```python
from build123d import *

# Parameters (mm, degrees)
F1_DEPTH = 30
F3_R     = 35
F4_DEPTH = 4
F5_D     = 9


with BuildPart() as f1:
    # F0 (on Right) → F1 (new body)
    with BuildSketch(Plane.YZ):
        with BuildLine():
            ThreePointArc((139.7, -30), (169.7, 0), (139.7, 30))
            Line((139.7, 30), (-139.7, 30))
            ThreePointArc((-139.7, 30), (-169.7, 0), (-139.7, -30))
            Line((-139.7, -30), (139.7, -30))
        make_face()
    extrude(amount=F1_DEPTH)

    # F3 (on mid) → F4 (cut, symmetric)
    with BuildSketch(Plane(origin=(15, 0, 0), x_dir=(0, -1, 0), z_dir=(-1, 0, 0))):
        with Locations((139.7, 0)):
            Circle(F3_R)
    extrude(amount=F4_DEPTH, both=True, mode=Mode.SUBTRACT)

    # F5 (through all)
    with Locations(Plane(origin=(0, 0, 0), x_dir=(0, 1, 0), z_dir=(-1, 0, 0))):
        with Locations((-139.7, 0)):
            Hole(F5_D / 2)


solid = f1.part
```
Source: CAD feature listing. Evaluate the final solid. Frame: model axes, mm. A direction names the side the tool comes from. Give positions to 0.01 mm unless a question says otherwise; leave off trailing zeros. Loops run counter-clockwise (first coordinate to the right, second up) from the corner with the lowest first, then second, coordinate; pieces in that order, holes last. Notation, with made-up numbers: (53.5, 64.25) - (109.5, 64.25) arc R28 ccw to (109.5, 94.25) - close; hole circle Ø7 at (87.25, 37.5). An arc over 180 degrees is marked (long way). Use CSV: the item, a comma, the result in double quotes. Start each with the question number.
1. Section A-A (z = 0). Output: boundary loops of the cut face in (x, y), then the cut area to 3 significant figures.
2. Draft query along Z for faces 3 (the cylindrical face through (14.79, 169.693, -0.66)), 4 (the cylindrical face through (24.58, -143.86, 1.72)), 5 (the flat face through (19, -137, 7)), 6 (the flat face through (30, -2, 0)). Return one class per face: +Z half, -Z half, draft (parallel to the pull), parting line (faces both ways), or undercut.
3. Reachability of faces 1 (the flat face through (15, 2, 30)), 2 (the flat face through (11, -137, 7)) from +Z, -Z, +X, -X, +Y, -Y: full face, straight path, thin tool, end or side. Return the list, or none.
4. Section B-B (x = 15.75). Output: boundary loops of the cut face in (y, z), then the cut area to 3 significant figures.
5. Pin query (flat end, axial travel): pin 1 (3 mm diameter, centred on x = 5.5, z = -1, fed in from +Y); pin 2 (8 mm diameter, centred on y = -139.7, z = 0, fed in from +X); pin 3 (2 mm diameter, centred on x = 15.5, z = -3.5, fed in from -Y). Return the tip coordinate at first contact, or that it passes through.
6. Section D-D (z = 24). Output: boundary loops of the cut face in (x, y), then the cut area to 3 significant figures.
7. Ray query, L1, parallel to Z at x = 26.5, y = -139.7; L2, parallel to X at y = -115, z = 2; L3, parallel to Y at x = 23, z = 21. Return the intervals inside material, ascending.
8. Section C-C (z = -21). Output: boundary loops of the cut face in (x, y), then the cut area to 3 significant figures.
Response:
1,outline,"(0, -169.7) - (11, -169.7) - (11, -144.2) - (0, -144.2) - close; (0, -135.2) - (11, -135.2) - (11, -104.7) - (19, -104.7) - (19, -135.2) - (30, -135.2) - (30, 169.7) - (0, 169.7) - close; (19, -169.7) - (30, -169.7) - (30, -144.2) - (19, -144.2) - close"
1,area,"9,460 mm²"
2,face 3,"parting line"
2,face 4,"undercut"
2,face 5,"undercut"
2,face 6,"draft"
3,face 1,"+Z, +X, -X, +Y, -Y"
3,face 2,"-Y"
4,outline,"(-121.67, -30) - (139.7, -30) arc R30 ccw to (139.7, 30) - (-121.67, 30) arc R35 cw to start"
4,area,"16,400 mm²"
5,pin 1,"y = 169.7"
5,pin 2,"through"
5,pin 3,"y = -104.99"
6,outline,"(0, -157.7) - (11, -157.7) - (11, -114.22) - (19, -114.22) - (19, -157.7) - (30, -157.7) - (30, 157.7) - (0, 157.7) - close"
6,area,"9,110 mm²"
7,L1,"-30 to -4.5, 4.5 to 30"
7,L2,"0 to 11, 19 to 30"
7,L3,"-161.12 to 161.12"
8,outline,"(0, -161.12) - (11, -161.12) - (11, -111.7) - (19, -111.7) - (19, -161.12) - (30, -161.12) - (30, 161.12) - (0, 161.12) - close"
8,area,"9,270 mm²"
